```python
from build123d import *

# Parameters (mm, degrees)
SKIZZE1_R                       = 22
SKIZZE1_R_2                     = 1.65
AUFSATZ_LINEAR_AUSTRAGEN1_DEPTH = 5
SKIZZE2_R                       = 2.9
SCHNITT_LINEAR_AUSTRAGEN1_DEPTH = 3
VERRUNDUNG1_SIZE                = 1


with BuildPart() as part:
    # Skizze1 → Aufsatz-Linear austragen1 (new body)
    with BuildSketch(Plane.XY):
        Circle(SKIZZE1_R)
        with Locations((10, 0)):
            Circle(SKIZZE1_R_2, mode=Mode.SUBTRACT)
        with Locations((0, -10)):
            Circle(SKIZZE1_R_2, mode=Mode.SUBTRACT)
        with Locations((-10, 0)):
            Circle(SKIZZE1_R_2, mode=Mode.SUBTRACT)
        with Locations((0, 10)):
            Circle(SKIZZE1_R_2, mode=Mode.SUBTRACT)
    extrude(amount=AUFSATZ_LINEAR_AUSTRAGEN1_DEPTH)

    # Skizze2 → Schnitt-Linear austragen1 (cut)
    with BuildSketch(Plane.XY.offset(5)):
        with Locations((0, 10)):
            Circle(SKIZZE2_R)
        with Locations((10, 0)):
            Circle(SKIZZE2_R)
        with Locations((0, -10)):
            Circle(SKIZZE2_R)
        with Locations((-10, 0)):
            Circle(SKIZZE2_R)
    extrude(amount=-SCHNITT_LINEAR_AUSTRAGEN1_DEPTH, mode=Mode.SUBTRACT)

    # Verrundung1
    verrundung1_edges = [part.edges().sort_by_distance(p)[0] for p in [
        (-2.9, 10, 5),
        (7.1, 0, 5),
        (-22, 0, 5),
        (-2.9, -10, 5),
        (-12.9, 0, 5),
    ]]
    chamfer(verrundung1_edges, length=VERRUNDUNG1_SIZE)


solid = part.part
```
Read the model definition and answer for the solid it produces. Units are mm, in the model's axes. A direction names the side the tool comes from. Coordinates: 2 decimals unless noted, no trailing zeros. Order: outer loops, then holes, each group sorted by start corner. A loop starts at its lowest first (then second) coordinate and runs counter-clockwise, first axis right, second up. Notation, with made-up numbers: (53, -19.5) - (78, -19.5) arc R18 ccw to (78, -13.5) - close; hole circle Ø11 at (12.5, 1.5). An arc over 180 degrees is marked (long way). Answer as a JSON object with one key per item and string values. Group by question number.
Item 1: Consider probe 1 along Y at (x, z) = (0, 0.8); probe 2 along Y at (x, z) = (0, 3.55); probe 3 along Z at (x, y) = (10, 2). Determine where each line is inside the solid, lowest interval first. Write a range as from..to.
Item 2: Section A-A (x = 0) is taken. Give the vertices of the cut face in (y, z).
Item 3: A tool of negligible diameter and unlimited length cuts with its end or side. For faces 5 (the face through (-0.4, 8.4, 1)), 6 (the face through (12, 0, 2)), from which of +Z, -Z, +X, -X, +Y, -Y can it reach the whole face along a straight path? Write none if from no direction.
Item 4: Flat-ended cylindrical pins translate along their axes: P1, Ø2, axis at x = 0, y = -10, coming from the +Z side; P2, Ø4.5, axis at x = -10.5, y = 0, coming from the +Z side; P3, Ø4.5, axis at x = 0, y = 10, coming from the -Z side; P4, Ø2, axis at x = -16.5, z = 3.5, coming from the -Y side. Find the tip coordinate at first contact, or state that the pin passes through.
Item 5: Section B-B (z = 1.5) is taken. Give the vertices of the cut face in (x, y), plus the area to 3 significant figures.
Item 6: The mould has two halves that part along X. Classify faces 1 (the face through (-8.476, -0.632, 0.986)), 2 (the face through (-2.9, -9.9, 3)), 3 (the face through (0, 0, 5)), 4 (the face through (-4.769, -21.477, 1.972)): +X half, -X half, draft (parallel to the pull), parting line (faces both ways), or undercut.
Results are:
{
 "1": {"probe 1": "y = -22..-11.65, -8.35..8.35, 11.65..22", "probe 2": "y = -22..-12.9, -7.1..7.1, 12.9..22", "probe 3": "z = 0..2"},
 "2": {"outline": "(-22, 0) - (-11.65, 0) - (-11.65, 2) - (-12.9, 2) - (-12.9, 4) - (-13.9, 5) - (-21, 5) - (-22, 4) - close; (-8.35, 0) - (8.35, 0) - (8.35, 2) - (7.1, 2) - (7.1, 4) - (6.1, 5) - (-6.1, 5) - (-7.1, 4) - (-7.1, 2) - (-8.35, 2) - close; (11.65, 0) - (22, 0) - (22, 4) - (21, 5) - (13.9, 5) - (12.9, 4) - (12.9, 2) - (11.65, 2) - close"},
 "3": {"face 5": "+Z, -Z", "face 6": "+Z"},
 "4": {"P1": "passes through", "P2": "stops at z = 2", "P3": "stops at z = 0", "P4": "stops at y = -15.61"},
 "5": {"outline": "circle Ø44 at (0, 0); hole circle Ø3.3 at (-10, 0); hole circle Ø3.3 at (0, -10); hole circle Ø3.3 at (0, 10); hole circle Ø3.3 at (10, 0)", "area": "1,490 mm^2"},
 "6": {"face 1": "undercut", "face 2": "undercut", "face 3": "draft", "face 4": "parting line"}
}
